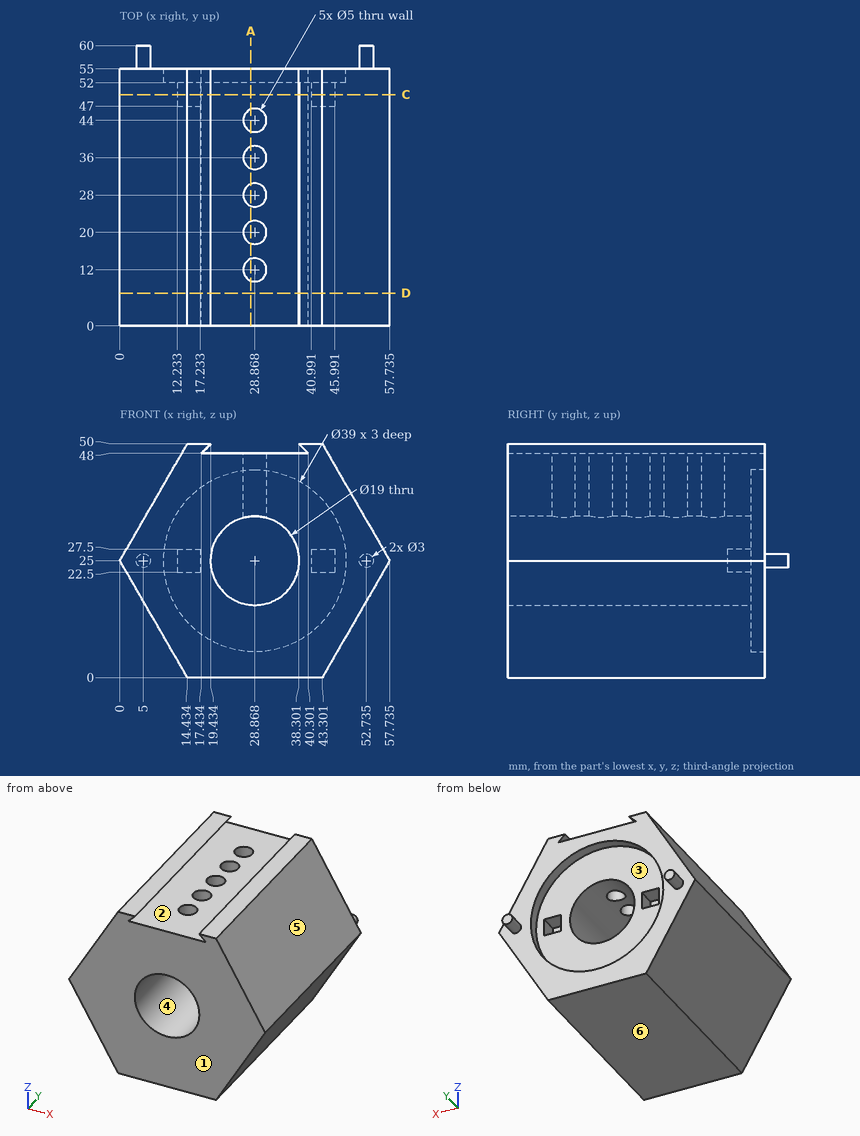
Drawing for the job (mm, zero at the part's lowest x, y, z). A direction names the side the tool comes from. Round coordinates to 2 decimals unless told otherwise and drop trailing zeros. Write each loop counter-clockwise with the first axis right and the second up, starting at its lowest first coordinate (ties: lowest second). Pieces come first, ordered by that corner, then holes. Notation, with made-up numbers: (-33.75, 77.25) - (23.25, 77.25) arc R20 ccw to (23.25, 92.25) - close; hole circle Ø4 at (-32.5, -27). An arc over 180 degrees is marked (long way). Use CSV: the item, a comma, the result in double quotes.
(1) Wall check: line 1 (Y direction, x = 45, z = 27); line 2 (Y direction, x = 42, z = 39); line 3 (X direction, y = 3, z = 28.5) (1 decimal). Give the ranges that are in metal, low to high.
Response:
line 1,"0 to 47"
line 2,"0 to 52"
line 3,"2 to 20, 37.7 to 55.7"
(2) Band-saw the part on C-C (y = 49.5). Write the cut outline in (x, z) (1 decimal), plus the area to 3 significant figures.
Response:
outline,"(0, 25) - (14.4, 0) - (43.3, 0) - (57.7, 25) - (43.3, 50) - (38.3, 50) - (40.3, 48) - (17.4, 48) - (19.4, 50) - (14.4, 50) - close; hole (12.2, 22.5) - (17.2, 22.5) - (17.2, 27.5) - (12.2, 27.5) - close; hole circle Ø19 at (28.9, 25); hole (41, 22.5) - (46, 22.5) - (46, 27.5) - (41, 27.5) - close"
area,"1,790 mm²"
(3) Band-saw the part on A-A (x = 28). Give the number of separate pieces and of enclosed holes in the cut face, plus the area to 3 significant figures.
Response:
separate pieces,"7"
enclosed holes,"0"
area,"1,220 mm²"
(4) Mould opens along X. For the marked faces 3, 4, 5 and 6 say: pulls with the +X half, pulls with the -X half, needs draft (parallel to the pull), parting line crosses it, or undercut.
Response:
face 3,"undercut"
face 4,"undercut"
face 5,"pulls with the +X half"
face 6,"needs draft"
(5) 3-axis set-ups, long thin cutter, end or side, ignore diameter. For the marked faces 1 and 2: which of +Z, -Z, +X, -X, +Y, -Y reach the whole face in a straight line?
Response:
face 1,"+Z, -Z, +X, -X, -Y"
face 2,"+Y, -Y"
(6) Band-saw the part on D-D (y = 7). Write the cut outline in (x, z) (1 decimal).
Response:
outline,"(0, 25) - (14.4, 0) - (43.3, 0) - (57.7, 25) - (43.3, 50) - (38.3, 50) - (40.3, 48) - (17.4, 48) - (19.4, 50) - (14.4, 50) - close; hole circle Ø19 at (28.9, 25)"
(7) Pin check, flat tips, straight feed: P1, Ø12, axis at x = 23, z = 19, coming from the +Y side; P2, Ø1.5, axis at x = 15, z = 26, coming from the +Y side; P3, Ø25, axis at x = 27.5, z = 32, coming from the +Y side. Stop position of each tip, or through.
Response:
P1,"y = 52"
P2,"y = 47"
P3,"y = 55"
